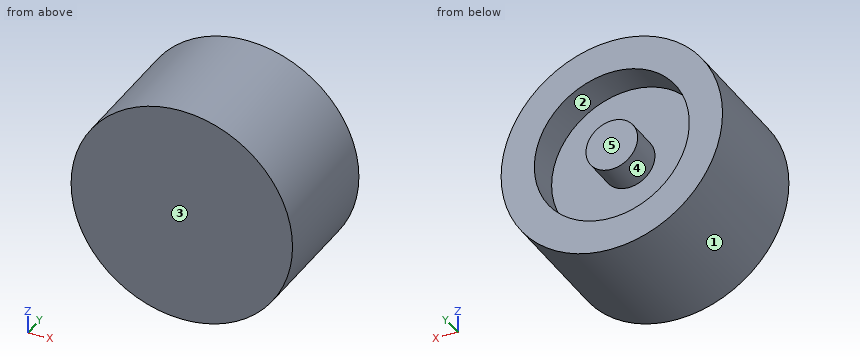
from build123d import *

# Parameters (mm, degrees)
CYLINDER003_R             = 3.5
CYLINDER003_DEPTH         = 10
CYLINDER002_R             = 10.5
CYLINDER002_DEPTH         = 5
CUT005007_PLACEMENT_ANGLE = 90
SKETCH005_R               = 15
EXTRUDE003002_DEPTH       = 17.25


with BuildPart() as cylinder003:
    # Cylinder003 → Cylinder003 (new body)
    with BuildSketch(Plane.XY.offset(-3)):
        Circle(CYLINDER003_R)
    extrude(amount=CYLINDER003_DEPTH)


with BuildPart() as obj1:
    # Cylinder002 → Cylinder002 (new body)
    with BuildSketch(Plane.XY):
        Circle(CYLINDER002_R)
    extrude(amount=CYLINDER002_DEPTH)

    # Cut005007: cut Cylinder003
    add(cylinder003.part, mode=Mode.SUBTRACT)


with BuildPart() as obj1_1:
    # Cut005007 placement: moved
    add(obj1.part.moved(Location((89, 0.5, 10.4))).rotate(Axis((89, 0.5, 10.4), (1, 0, 0)), CUT005007_PLACEMENT_ANGLE))


with BuildPart() as cut005008:
    # Sketch005 → Extrude003002 (new body)
    with BuildSketch(Plane.XZ):
        with Locations((89, 10.4)):
            Circle(SKETCH005_R)
    extrude(amount=EXTRUDE003002_DEPTH)

    # Cut005008: cut obj1
    add(obj1_1.part, mode=Mode.SUBTRACT)


solid = cut005008.part
Can you work these out from the model? Positions are in its coordinate system, mm. Face numbers are marked on the shaded views. A direction names the side the tool comes from. Coordinates: 2 decimals unless noted, no trailing zeros. Order: outer loops, then holes, each group sorted by start corner. A loop starts at its lowest first (then second) coordinate and runs counter-clockwise, first axis right, second up. Notation, with made-up numbers: M 73,-37 L 125,-37 A16 cw 125,-21 Z; hole C -33,68.25 d9. An arc over 180 degrees is marked long. Answer as CSV lines item,"result".
(1) Please list where these lines run through material, in increasing order: L1, parallel to Z at x = 89, y = -3.05; L2, parallel to Z at x = 86.5, y = -4.25; L3, parallel to Y at x = 93.25, z = 15.75.
Geometry check:
L1,"-4.6 to -0.1, 6.9 to 13.9, 20.9 to 25.4"
L2,"-4.39 to 0.2, 7.95 to 12.85, 20.6 to 25.19"
L3,"-17.25 to -4.5"
(2) Suppose I cut it at A-A on z = 10.4. Please give me the cut outline in (x, y), plus the area to 4 significant figures.
Geometry check:
outline,"M 74,-17.25 L 104,-17.25 L 104,0 L 99.5,0 L 99.5,-4.5 L 92.5,-4.5 L 92.5,0 L 85.5,0 L 85.5,-4.5 L 78.5,-4.5 L 78.5,0 L 74,0 Z"
area,"454.5 mm^2"
(3) On a 3-axis mill with a long thin cutter (end or side, diameter ignored), from which of +Z, -Z, +X, -X, +Y, -Y can I reach the whole of each face in a straight line? I mean the marked faces 4 and 5. Say none if no direction works.
Geometry check:
face 4,"+Y"
face 5,"+Z, -Z, +X, -X, +Y"
(4) I'm going to push flat-ended pins straight in: pin 1 (10 mm diameter, centred on x = 81.5, z = 11.5, fed in from +Y); pin 2 (8 mm diameter, centred on x = 98, y = -2, fed in from -Z); pin 3 (1.5 mm diameter, centred on x = 84, y = -15, fed in from -Z); pin 4 (4 mm diameter, centred on y = -14.5, z = 7, fed in from -X). Where does each tip first touch, or does it pass through?
Geometry check:
pin 1,"y = 0"
pin 2,"z = -3.74"
pin 3,"z = -3.99"
pin 4,"x = 74.07"
(5) If we mould it in two halves opening along Z, with no side actions, what happens to the marked faces 1, 2 and 3? For each: released by +Z, released by -Z, zero draft, split by the parting line, or undercut.
Geometry check:
face 1,"split by the parting line"
face 2,"undercut"
face 3,"zero draft"
(6) Suppose I cut it at C-C on x = 89. Please give me the cut outline in (y, z).
Geometry check:
outline,"M -17.25,-4.6 L 0,-4.6 L 0,-0.1 L -4.5,-0.1 L -4.5,6.9 L 0,6.9 L 0,13.9 L -4.5,13.9 L -4.5,20.9 L 0,20.9 L 0,25.4 L -17.25,25.4 Z"
(7) Suppose I cut it at B-B on y = -4. Please give me the cut outline in (x, z).
Geometry check:
outline,"C 89,10.4 d30; C 89,10.4 d7; hole C 89,10.4 d21"
(8) Suppose I cut it at D-D on z = 16.25. Please give me the cut outline in (x, y), plus the area to 3 significant figures.
Geometry check:
outline,"M 75.19,-17.25 L 102.81,-17.25 L 102.81,0 L 97.72,0 L 97.72,-4.5 L 80.28,-4.5 L 80.28,0 L 75.19,0 Z"
area,"398 mm^2"
